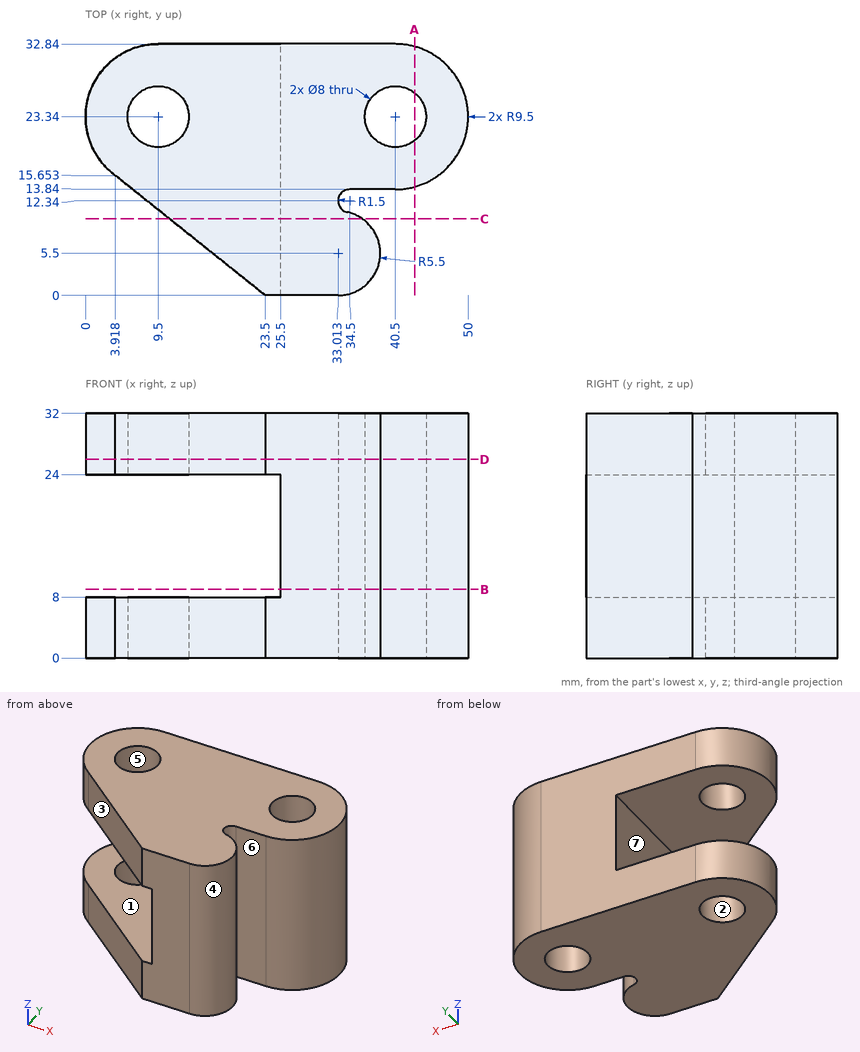
The figure shows three views and two pictorial views of one solid part (mm, origin at its lowest corner). Answer the questions. A direction names the side the tool comes from. Coordinates: 2 decimals unless noted, no trailing zeros. Order: outer loops, then holes, each group sorted by start corner. A loop starts at its lowest first (then second) coordinate and runs counter-clockwise, first axis right, second up.
Q1. A cutting plane is placed at B-B, the plane z = 9. Write down the section's boundary in (x, y), and give its area (3 significant figures).
Q2. A cutting plane is placed at A-A, the plane x = 43. Write down the section's boundary in (y, z) (1 decimal).
Q3. A cutting plane is placed at C-C, the plane y = 10. Write down the section's boundary in (x, z) (1 decimal).
Q4. A cutting plane is placed at D-D, the plane z = 26. Write down the section's boundary in (x, y).
Q5. For a pull along X with two mould halves and no side action, classify the marked faces 1, 2, 3 and 4 as pulls with the +X half, pulls with the -X half, needs draft (parallel to the pull), parting line crosses it, or undercut.
Q6. Given P1, Ø5, axis at y = 13.5, z = 13.5, coming from the -X side; P2, Ø5, axis at x = 9.5, y = 23.34, coming from the -Z side; P3, Ø6.5, axis at x = 37, z = 18, coming from the -Y side; P4, Ø5, axis at x = 43, z = 14.5, coming from the -Y side, each flat-ended and moving along its own axis, determine where each tip first touches the part or whether it passes through.
Q7. Consider line 1 (Z direction, x = 18, y = 21.5); line 2 (X direction, y = 26.5, z = 4); line 3 (Y direction, x = 9, z = 27). Determine where each line is inside the solid, lowest interval first.
Q8. Which of the six approach directions +Z, -Z, +X, -X, +Y, -Y give full straight-line access (tool end or side, diameter ignored) to the marked faces 5, 6 and 7?
Answers follow:
1. outline: (25.5, 0) - (33.01, 0) arc R5.5 ccw to (34.18, 10.87) arc R1.5 cw to (34.5, 13.84) - (40.5, 13.84) arc R9.5 ccw to (40.5, 32.84) - (25.5, 32.84) - close; hole circle Ø8 at (40.5, 23.34)
1. area: 529 mm2
2. outline: (14.2, 0) - (20.2, 0) - (20.2, 32) - (14.2, 32) - close; (26.5, 0) - (32.5, 0) - (32.5, 32) - (26.5, 32) - close
3. outline: (11, 0) - (36.2, 0) - (36.2, 32) - (11, 32) - (11, 24) - (25.5, 24) - (25.5, 8) - (11, 8) - close
4. outline: (3.92, 15.65) - (23.5, 0) - (33.01, 0) arc R5.5 ccw to (34.18, 10.87) arc R1.5 cw to (34.5, 13.84) - (40.5, 13.84) arc R9.5 ccw to (40.5, 32.84) - (9.5, 32.84) arc R9.5 ccw to start; hole circle Ø8 at (9.5, 23.34); hole circle Ø8 at (40.5, 23.34)
5. face 1: needs draft
5. face 2: undercut
5. face 3: pulls with the -X half
5. face 4: pulls with the +X half
6. P1: stops at x = 25.5
6. P2: passes through
6. P3: stops at y = 0.05
6. P4: stops at y = 13.84
7. line 1: z = 0 to 8, 24 to 32
7. line 2: x = 0.54 to 7.05, 11.95 to 38.05, 42.95 to 49.46
7. line 3: y = 11.59 to 19.37, 27.31 to 32.83
8. face 5: +Z, -Z
8. face 6: +Z, -Z, +X
8. face 7: -X, +Y, -Y
